Autodesk Fusion 360 part; units mm, degrees
sketch "草图1" plane through (0, 0, 0) normal (1, 0, 0) x (0, 1, 0)
  circle A0 centre (0, 0) radius 15
  circle A1 centre (0, 0) radius 9
  line L0 (0, 15) -> (-40, 15)
  line L1 (-40, 15) -> (-40, 6)
  line L2 (-40, 6) -> (-20, 6)
  line L3 (-20, 6) -> (-20, -6)
  line L4 (-20, -6) -> (-40, -6)
  line L5 (-40, -6) -> (-40, -15)
  line L6 (-40, -15) -> (0, -15)
  line L7 (-157.7005, 0) -> (55, 0) construction
  dimension "d1" = 30
  dimension "d2" = 18
  dimension "d3" = 12
  dimension "d4" = 20
  dimension "d5" = 40
extrude "拉伸1" add sketch "草图1" along normal mid plane 48 contours A0
extrude "拉伸2" add sketch "草图1" along normal mid plane 42 contours A0 L0 L1 L2 L3 L4 L5 L6
fillet "圆角1" radius 10 4 edges at (21, -40, 10.5) (21, -40, -10.5) (-21, -40, 10.5) (-21, -40, -10.5)
sketch "草图2" plane through (0, 0, 15) normal (0, 0, 1) x (-1, 0, 0)
  arc A0 (21, 30) -> (11, 40) centre (11, 30) ccw
  line L0 (11, 40) -> (-11, 40)
  arc A1 (-11, 40) -> (-21, 30) centre (-11, 30) ccw
  line L1 (-21, 30) -> (-21, 0)
  line L2 (-21, 0) -> (21, 0)
  line L3 (21, 0) -> (21, 30)
  line L4 (21, 30) -> (-21, 30)
  circle A2 centre (11, 30) radius 4
  circle A3 centre (-11, 30) radius 4
  line L5 (0, 0) -> (0, 40)
  line L6 (-11, 30) -> (-11, 40)
  dimension "d12" = 8
extrude "拉伸3" cut sketch "草图2" against normal through all contours L4 A2 | L4 A2 | L4 A3 L6 | L4 A3 L6 | L4 A3
The listing builds one solid part. Answer for the finished solid, in the listing's coordinates (mm). A direction names the side the tool comes from. Give positions to 0.01 mm unless a question says otherwise; leave off trailing zeros. Write each loop counter-clockwise with the first axis right and the second up, starting at its lowest first coordinate (ties: lowest second). Pieces come first, ordered by that corner, then holes. Notation, with made-up numbers: (63, -39.75) - (74, -39.75) arc R27 ccw to (74, -10.75) - close; hole circle Ø9 at (85.25, -28). An arc over 180 degrees is marked (long way). Use one line per item in the form item = value. Start each with the question number.
1) The mould has two halves that part along Y. Classify faces 1 (the face through (0, -20, 0)), 2 (the face through (-10.479, -33.966, 10.563)), 3 (the face through (0, -30, 6)), 4 (the face through (11.521, -33.966, 10.563)): pulls with the +Y half, pulls with the -Y half, needs draft (parallel to the pull), parting line crosses it, or undercut.
2) Find section A-A on x = -8. Determine the outline of the cut face in (y, z).
3) Flat-ended cylindrical pins translate along their axes: pin 1 Ø7 at (x, y) = (11, -30) entering from -Z; pin 2 Ø12 at (x, z) = (-17.5, -10) entering from -Y; pin 3 Ø1.5 at (y, z) = (-19, 9.5) entering from +X; pin 4 Ø8 at (x, z) = (12.5, 0) entering from -Y. Find the tip coordinate at first contact, or state that the pin passes through.
4) Find section D-D on z = 0. Determine the outline of the cut face in (x, y).
5) Find section C-C on x = 5.5. Determine the outline of the cut face in (y, z).
6) Find section B-B on z = 7. Determine the outline of the cut face in (x, y), plus the area to 3 significant figures.
7) A tool of negligible diameter and unlimited length cuts with its end or side. For faces 5 (the face through (0, -40, 11)), 6 (the face through (0, -30, -6)), from which of +Z, -Z, +X, -X, +Y, -Y can it reach the whole face along a straight path? Write none if from no direction.
8) Consider line 1 along X through (y, z) = (-30, -8.5); line 2 along Z through (x, y) = (-17, -25); line 3 along Z through (x, y) = (9, 0). Determine where each line is inside the solid, lowest interval first. Write a range as from..to.
Geometry results:
q1.face_1 = pulls with the -Y half
q1.face_2 = undercut
q1.face_3 = needs draft
q1.face_4 = undercut
q2.outline = (-40, -15) - (-32.65, -15) - (-32.65, -6) - (-40, -6) - close; (-40, 6) - (-32.65, 6) - (-32.65, 15) - (-40, 15) - close; (-27.35, -15) - (0, -15) arc R15 ccw to (0, 15) - (-27.35, 15) - (-27.35, 6) - (-20, 6) - (-20, -6) - (-27.35, -6) - close; hole circle Ø18 at (0, 0)
q3.pin_1 = through
q3.pin_2 = -39.99
q3.pin_3 = 21
q3.pin_4 = -20
q4.outline = (-24, -15) - (-21, -15) - (-21, -20) - (21, -20) - (21, -15) - (24, -15) - (24, -9) - (-24, -9) - close; (-24, 9) - (24, 9) - (24, 15) - (-24, 15) - close
q5.outline = (-40, -15) - (0, -15) arc R15 ccw to (0, 15) - (-40, 15) - (-40, 6) - (-20, 6) - (-20, -6) - (-40, -6) - close; hole circle Ø18 at (0, 0)
q6.outline = (-24, -13.27) - (-21, -13.27) - (-21, -30) arc R10 ccw to (-11, -40) - (11, -40) arc R10 ccw to (21, -30) - (21, -13.27) - (24, -13.27) - (24, -5.66) - (-24, -5.66) - close; (-24, 5.66) - (24, 5.66) - (24, 13.27) - (-24, 13.27) - close; hole circle Ø8 at (-11, -30); hole circle Ø8 at (11, -30)
q6.area = 1,710 mm2
q7.face_5 = +Z, -Z, +X, -X, -Y
q7.face_6 = +X, -X, -Y
q8.line_1 = -21..-15, -7..7, 15..21
q8.line_2 = -15..-6, 6..15
q8.line_3 = -15..-9, 9..15
